Build history of the part. All positions in model axes, mm. Face numbers are marked on the shaded views. A direction names the side the tool comes from. Give positions to 0.01 mm unless a question says otherwise; leave off trailing zeros. Put each result on its own line as item: value.
from build123d import *

# Parameters (mm, degrees)
SKETCH1_R                = 3.25
BOSS_EXTRUDE1_DEPTH      = 4
BOSS_EXTRUDE4_DEPTH      = 0.4
FILLET1_R                = 2
CIRPATTERN2_COUNT        = 3
FILLET1_OF_CIRPATTERN2_R = 2
CUT_EXTRUDE1_REACH       = 23.637
FILLET2_R                = 0.3


with BuildPart() as part:
    # Sketch1 → Boss-Extrude1 (new, symmetric)
    with BuildSketch(Plane.XY):
        Circle(SKETCH1_R)
    extrude(amount=BOSS_EXTRUDE1_DEPTH, both=True)

    # Sketch6 → Boss-Extrude4 (add, symmetric)
    with BuildSketch(Plane(origin=(0, 0, 0), x_dir=(-1, 0, 0), z_dir=(0, 0.866025403784438, -0.500000000000001))):
        with BuildLine():
            Line((0, 0), (-10, 8))
            ThreePointArc((-10, 8), (-14, 0), (-10, -8))
            Line((-10, -8), (0, 0))
        make_face()
    boss_extrude4 = extrude(amount=BOSS_EXTRUDE4_DEPTH, both=True)

    # Fillet1
    fillet1_edges = [part.edges().sort_by_distance(p)[0] for p in [
        (10, 4, 6.92820323),
        (10, -4, -6.92820323),
    ]]
    fillet(fillet1_edges, radius=FILLET1_R)

    # CirPattern2: Boss-Extrude4 ×3 about axis
    cirpattern2_axis = Axis((0, 0, 0), (0, 0, 1))
    for i in range(1, CIRPATTERN2_COUNT):
        add(boss_extrude4.rotate(cirpattern2_axis, i * 360 / CIRPATTERN2_COUNT))

    # Fillet1 of CirPattern2
    fillet1_of_cirpattern2_edges = [part.edges().sort_by_distance(p)[0] for p in [
        (-8.464101615, 6.660254038, 6.92820323),
        (-1.535898385, 10.660254038, -6.92820323),
        (-1.535898385, -10.660254038, 6.92820323),
        (-8.464101615, -6.660254038, -6.92820323),
    ]]
    fillet(fillet1_of_cirpattern2_edges, radius=FILLET1_OF_CIRPATTERN2_R)

    # Sketch7 → Cut-Extrude1 (cut, up to next)
    with BuildSketch(Plane.XY.offset(4), mode=Mode.PRIVATE) as cut_extrude1_sk1:
        with BuildLine():
            Line((1.484313483, 2.011669328), (0.366025404, 1.366025404))
            Line((0.366025404, 1.366025404), (-0.27961852, 2.484313483))
            ThreePointArc((-0.27961852, 2.484313483), (-1.25, 2.165063509), (-2.011669328, 1.484313483))
            Line((-2.011669328, 1.484313483), (-1.366025404, 0.366025404))
            Line((-1.366025404, 0.366025404), (-2.484313483, -0.27961852))
            ThreePointArc((-2.484313483, -0.27961852), (-2.165063509, -1.25), (-1.484313483, -2.011669328))
            Line((-1.484313483, -2.011669328), (-0.366025404, -1.366025404))
            Line((-0.366025404, -1.366025404), (0.27961852, -2.484313483))
            ThreePointArc((0.27961852, -2.484313483), (1.25, -2.165063509), (2.011669328, -1.484313483))
            Line((2.011669328, -1.484313483), (1.366025404, -0.366025404))
            Line((1.366025404, -0.366025404), (2.484313483, 0.27961852))
            ThreePointArc((2.484313483, 0.27961852), (2.165063509, 1.25), (1.484313483, 2.011669328))
        make_face()
    cut_extrude1_tool1 = extrude(cut_extrude1_sk1.sketch, amount=-CUT_EXTRUDE1_REACH, mode=Mode.PRIVATE) & part.part
    add(cut_extrude1_tool1.solids().sort_by_distance((0, 0, 4))[0], mode=Mode.SUBTRACT)

    # Fillet2
    fillet2_edges = [part.edges().sort_by_distance(p)[0] for p in [
        (-1.20587358, -6.114217695, 4.286257479),
        (-2.149245107, -10.400789842, 6.583480561),
        (-7.3, -11.951150572, 0.2),
        (-8.532725669, -6.715285621, -6.183480561),
        (-0.587527, -6.333289225, 3.803498858),
        (-1.549245107, -10.747200003, 6.183480561),
        (-6.7, -12.297560734, -0.2),
        (-7.932725669, -7.061695783, -6.583480561),
        (-5.191025858, 3.67545792, 3.803498858),
        (-8.532725669, 6.715285621, 6.183480561),
        (-7.3, 11.951150572, -0.2),
        (-1.20587358, 6.114217695, -4.286257479),
        (-0.587527, 6.333289225, -3.803498858),
        (-4.692131059, 4.101426001, 4.286257479),
        (-7.932725669, 7.061695783, 6.583480561),
        (-6.7, 12.297560734, 0.2),
        (5.778552858, -2.657831305, -3.803498858),
        (10.081970776, -4.031914382, -6.183480561),
        (14, -0.346410162, 0.2),
        (10.081970776, 3.339094059, 6.583480561),
        (5.898004638, -2.012791694, -4.286257479),
        (10.081970776, -3.339094059, -6.583480561),
        (14, 0.346410162, -0.2),
        (10.081970776, 4.031914382, 6.183480561),
        (-5.191025858, -3.67545792, -3.803498858),
        (-4.692131059, -4.101426001, -4.286257479),
        (-2.149245107, 10.400789842, -6.583480561),
        (-1.549245107, 10.747200003, -6.183480561),
        (5.898004638, 2.012791694, 4.286257479),
        (5.778552858, 2.657831305, 3.803498858),
    ]]
    fillet(fillet2_edges, radius=FILLET2_R)


solid = part.part
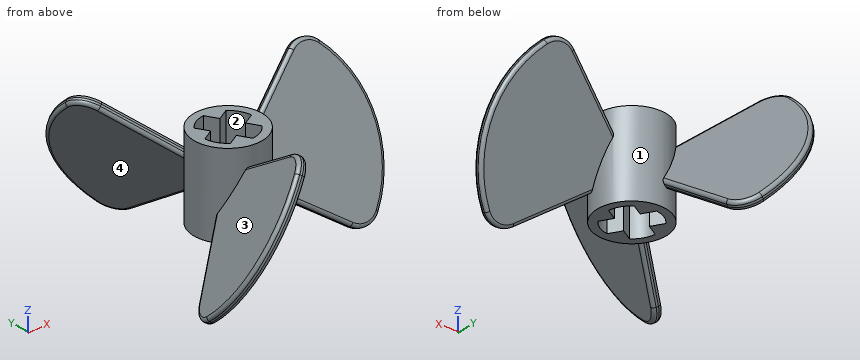
1) Slice it at A-A (z = -3). Give the number of separate pieces and of enclosed holes in the cut face, plus the area to 3 significant figures.
Filled sheet:
separate pieces: 4
enclosed holes: 1
area: 42.5 mm2
2) Pin check, flat tips, straight feed: pin 1 (6 mm diameter, centred on x = -6, y = 0.5, fed in from -Z); pin 2 (5 mm diameter, centred on x = -5, z = 4.5, fed in from +Y); pin 3 (2 mm diameter, centred on y = -7, z = 4, fed in from +X); pin 4 (10 mm diameter, centred on x = -5.5, y = 7, fed in from +Z). Stop position of each tip, or through.
Filled sheet:
pin 1: z = -4
pin 2: y = 9.59
pin 3: x = -0.67
pin 4: z = 6.48
3) Tool access for the marked faces 1, 2, 3 and 4: list every direction of +Z, -Z, +X, -X, +Y, -Y with a clear straight run to the whole face (end or side of a thin tool).
Filled sheet:
face 1: none
face 2: +Z, -Z
face 3: +Z, -X
face 4: -Z, -X
4) Wall check: L1, parallel to X at y = -0.75, z = 2.75; L2, parallel to Z at x = -7.25, y = -6.25; L3, parallel to Y at x = -5.5, z = 2. Give the ranges that are in metal, low to high.
Filled sheet:
L1: -3.16 to -2.38, 1.59 to 3.16
L2: -6.22 to -4.66
L3: -12.53 to -10.91, 6.29 to 8.14
